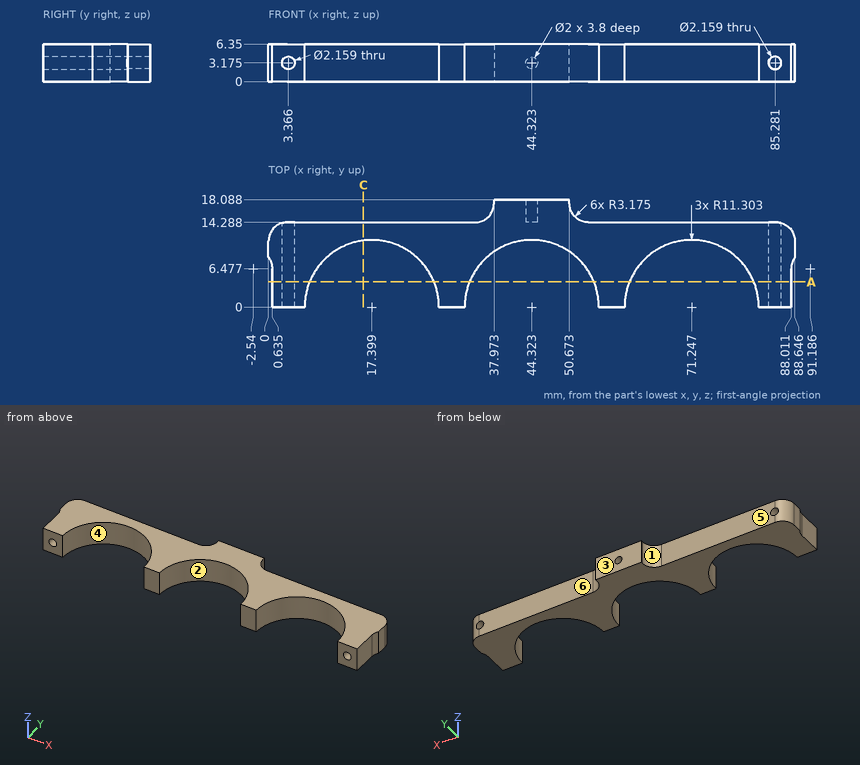
For this review, use the dimensioned drawing (mm, ordinates from the lowest corner) and the shaded views. A direction names the side the tool comes from. Coordinates: 2 decimals unless noted, no trailing zeros. Order: outer loops, then holes, each group sorted by start corner. A loop starts at its lowest first (then second) coordinate and runs counter-clockwise, first axis right, second up. Notation, with made-up numbers: (41.25, -6) -> (89.25, -6) arc R27 ccw to (89.25, 15) -> close; hole circle Ø10 at (68.25, -20). An arc over 180 degrees is marked (long way). One line per item, written item: value. Start each with the question number.
Q1. Mouldability with a two-part tool opening along X and no side actions: class the marked faces 1, 2 and 3 as pulls with the +X half, pulls with the -X half, needs draft (parallel to the pull), parting line crosses it, or undercut.
Q2. For probe 1 along X at (y, z) = (6, 1.5) (1 decimal); probe 2 along X at (y, z) = (2, 2) (1 decimal); probe 3 along X at (y, z) = (9, 3) (1 decimal), list the stretches that pass through material, from the lowest coordinate up.
Q3. Take a section at A-A, the plane y = 4.25. Give the number of separate pieces and of enclosed holes in the cut face.
Q4. Take a section at C-C, the plane x = 16. State the section outline as (y, z) points.
Q5. Insertion check: pin 1 Ø1.9 at (y, z) = (1.5, 1.5) entering from -X (1 decimal); pin 2 Ø1.5 at (x, z) = (65, 2.5) entering from +Y; pin 3 Ø3 at (y, z) = (2, 4.5) entering from +X. Each pin has a flat end and moves straight along its axis. Give the tip position at first contact, or say it passes through.
Q6. Tool access review of the marked faces 4, 5 and 6: name each direction out of +Z, -Z, +X, -X, +Y, -Y from which nothing blocks a thin tool from reaching the whole face with its end or side.
Values follow:
1. face 1: pulls with the -X half
1. face 2: undercut
1. face 3: needs draft
2. probe 1: x = 0.6 to 7.8, 27 to 34.7, 53.9 to 61.7, 80.8 to 88
2. probe 2: x = 0.6 to 6.3, 28.5 to 33.2, 55.4 to 60.1, 82.4 to 88
2. probe 3: x = 0 to 2.3, 4.4 to 10.6, 24.2 to 37.5, 51.2 to 64.4, 78.1 to 84.2, 86.3 to 88.6
3. separate pieces: 4
3. enclosed holes: 2
4. outline: (11.22, 0) -> (14.29, 0) -> (14.29, 6.35) -> (11.22, 6.35) -> close
5. pin 1: stops at x = 0.6
5. pin 2: stops at y = 14.29
5. pin 3: stops at x = 88.01
6. face 4: +Z, -Z, -Y
6. face 5: +Z, -Z, -X, +Y
6. face 6: +Z, -Z, +X, +Y
